from build123d import *

# Parameters (mm, degrees)
SKETCH1_W                      = 125
SKETCH1_H                      = 290
BASE_FLANGE1_DEPTH             = 3.03784
EDGE_FLANGE1_DEPTH             = 290
EDGE_FLANGE1_BEND_DEPTH        = 290
EDGE_FLANGE2_STRIP_W           = 18.50136
EDGE_FLANGE2_STRIP_H           = 3.03784
EDGE_FLANGE2_STRIP_CUT_DEPTH   = 290
EDGE_FLANGE2_STRIP_2_W         = 18.50136
EDGE_FLANGE2_STRIP_2_H         = 3.03784
EDGE_FLANGE2_STRIP_CUT_2_DEPTH = 290
EDGE_FLANGE2_DEPTH             = 290
EDGE_FLANGE2_BEND_DEPTH        = 290
M6_CLEARANCE_HOLE1_D           = 8
CUT_EXTRUDE1_DEPTH             = 50


# Sheet-metal steps are written as plain solids
with BuildPart() as part:
    # Sketch1 → Base-Flange1 (new body)
    with BuildSketch(Plane(origin=(0, 0, 0), x_dir=(0, 0, -1), z_dir=(1, 0, 0))):
        Rectangle(SKETCH1_W, SKETCH1_H)
    extrude(amount=-BASE_FLANGE1_DEPTH)

    # Edge-Flange1 section (across the edge) → Edge-Flange1 (add)
    with BuildSketch(Plane(origin=(-3.03784, -145, 65.675), x_dir=(0, 0, -1), z_dir=(0, 1, 0))):
        with BuildLine():
            Line((-3.03784, 3.175), (-3.03784, 55))
            Line((-3.03784, 55), (0, 55))
            Line((0, 55), (0, 3.175))
            ThreePointArc((0, 3.175), (0.92993597, 0.92993597), (3.175, 0))
            Line((3.175, 0), (3.175, -3.03784))
            ThreePointArc((3.175, -3.03784), (-1.218141294, -1.218141294), (-3.03784, 3.175))
        make_face()
    extrude(amount=EDGE_FLANGE1_DEPTH)

    # Edge-Flange1 section 2 (across the edge) → Edge-Flange1 bend (add)
    with BuildSketch(Plane(origin=(-3.03784, 145, -65.675), x_dir=(0, 0, 1), z_dir=(0, -1, 0))):
        with BuildLine():
            Line((-3.03784, 3.175), (-3.03784, 55))
            Line((-3.03784, 55), (0, 55))
            Line((0, 55), (0, 3.175))
            ThreePointArc((0, 3.175), (0.92993597, 0.92993597), (3.175, 0))
            Line((3.175, 0), (3.175, -3.03784))
            ThreePointArc((3.175, -3.03784), (-1.218141294, -1.218141294), (-3.03784, 3.175))
        make_face()
    extrude(amount=EDGE_FLANGE1_BEND_DEPTH)

    # Edge-Flange2 strip (across the edge) → Edge-Flange2 strip cut (cut)
    with BuildSketch(Plane(origin=(-58.03784, -145, -68.71284), x_dir=(1, 0, 0), z_dir=(0, 1, 0))):
        with Locations((-3.03784, -1.51892)):
            Rectangle(EDGE_FLANGE2_STRIP_W, EDGE_FLANGE2_STRIP_H)
    extrude(amount=EDGE_FLANGE2_STRIP_CUT_DEPTH, mode=Mode.SUBTRACT)

    # Edge-Flange2 strip 2 (across the edge) → Edge-Flange2 strip cut 2 (cut)
    with BuildSketch(Plane(origin=(-58.03784, 145, 68.71284), x_dir=(1, 0, 0), z_dir=(0, -1, 0))):
        with Locations((-3.03784, -1.51892)):
            Rectangle(EDGE_FLANGE2_STRIP_2_W, EDGE_FLANGE2_STRIP_2_H)
    extrude(amount=EDGE_FLANGE2_STRIP_CUT_2_DEPTH, mode=Mode.SUBTRACT)

    # Edge-Flange2 section (across the edge) → Edge-Flange2 (add)
    with BuildSketch(Plane(origin=(-58.03784, -145, -68.71284), x_dir=(1, 0, 0), z_dir=(0, 1, 0))):
        with BuildLine():
            Line((0, 3.175), (0, 30))
            Line((0, 30), (3.03784, 30))
            Line((3.03784, 30), (3.03784, 3.175))
            ThreePointArc((3.03784, 3.175), (3.96777597, 0.92993597), (6.21284, 0))
            Line((6.21284, 0), (6.21284, -3.03784))
            ThreePointArc((6.21284, -3.03784), (1.819698706, -1.218141294), (0, 3.175))
        make_face()
    extrude(amount=EDGE_FLANGE2_DEPTH)

    # Edge-Flange2 section 2 (across the edge) → Edge-Flange2 bend (add)
    with BuildSketch(Plane(origin=(-58.03784, 145, 68.71284), x_dir=(1, 0, 0), z_dir=(0, -1, 0))):
        with BuildLine():
            Line((0, 3.175), (0, 30))
            Line((0, 30), (3.03784, 30))
            Line((3.03784, 30), (3.03784, 3.175))
            ThreePointArc((3.03784, 3.175), (3.96777597, 0.92993597), (6.21284, 0))
            Line((6.21284, 0), (6.21284, -3.03784))
            ThreePointArc((6.21284, -3.03784), (1.819698706, -1.218141294), (0, 3.175))
        make_face()
    extrude(amount=EDGE_FLANGE2_BEND_DEPTH)

    # M6 Clearance Hole1 (through all)
    with Locations(Plane(origin=(-55, 0, 0), x_dir=(0, 0, -1), z_dir=(1, 0, 0))):
        with Locations((-80, 120), (80, 120), (80, -120), (-80, -120)):
            Hole(M6_CLEARANCE_HOLE1_D / 2)

    # Sketch20 → Cut-Extrude1 (cut)
    with BuildSketch(Plane.XY.offset(98.71284)):
        with BuildLine():
            Line((-58.03784, 56.1), (-32.63784, 56.1))
            ThreePointArc((-32.63784, 56.1), (-19.93784, 43.4), (-32.63784, 30.7))
            Line((-32.63784, 30.7), (-58.03784, 30.7))
            Line((-58.03784, 30.7), (-58.03784, 56.1))
        make_face()
    extrude(amount=-CUT_EXTRUDE1_DEPTH, mode=Mode.SUBTRACT)


solid = part.part
Here's how the part is built. I have some questions about the finished solid (model axes, mm). A direction names the side the tool comes from. Coordinates: 2 decimals unless noted, no trailing zeros. Order: outer loops, then holes, each group sorted by start corner. A loop starts at its lowest first (then second) coordinate and runs counter-clockwise, first axis right, second up. Notation, with made-up numbers: (12.25, 59) -> (46.25, 59) arc R30 ccw to (46.25, 98) -> close; hole circle Ø9 at (15.5, 13.25). An arc over 180 degrees is marked (long way). Answer in a Markdown table with one row per item.
(1) I want a section at D-D on z = -80. List the corners of the cut face in (x, y) for me.
Answer key:
| item | result |
|---|---|
| outline | (-58.04, -145) -> (-55, -145) -> (-55, -124) -> (-58.04, -124) -> close; (-58.04, -116) -> (-55, -116) -> (-55, 116) -> (-58.04, 116) -> close; (-58.04, 124) -> (-55, 124) -> (-55, 145) -> (-58.04, 145) -> close |
(2) On a 3-axis mill with a long thin cutter (end or side, diameter ignored), from which of +Z, -Z, +X, -X, +Y, -Y can I reach the whole of each face in a straight line? I mean faces 1 (the face through (-55, 101, 85)), 2 (the face through (-3.038, 2, 1)), 3 (the face through (-56, 30.7, 76)), 4 (the face through (0, 2, 1)), 5 (the face through (-29, 2, -68.713)). Say none if no direction works.
Answer key:
| item | result |
|---|---|
| face 1 | +Z, +X, +Y, -Y |
| face 2 | -X, +Y, -Y |
| face 3 | +Z, -X |
| face 4 | +Z, -Z, +X, +Y, -Y |
| face 5 | -Z, +X, +Y, -Y |
(3) Thinking about a two-plate mould opening in Y: for faces 6 (the face through (-56.54, 123.966, 79.479)), 7 (the face through (-58.038, -56, 85)), 8 (the face through (-1, 145, 30)), which applies, +Y half, -Y half, draft (parallel to the pull), parting line (faces both ways), or undercut?
Answer key:
| item | result |
|---|---|
| face 6 | undercut |
| face 7 | draft |
| face 8 | +Y half |
(4) Will these pins go through, and if not, where does the flat tip stop? pin 1 Ø13.5 at (y, z) = (98, 86.5) entering from +X; pin 2 Ø4 at (x, y) = (-35, 69) entering from -Z; pin 3 Ø10 at (x, z) = (-12, 55.5) entering from -Y; pin 4 Ø23 at (x, y) = (-22, -4) entering from +Z.
Answer key:
| item | result |
|---|---|
| pin 1 | x = -55 |
| pin 2 | z = -68.71 |
| pin 3 | through |
| pin 4 | z = 68.71 |
(5) I want a section at C-C on y = 78. List the corners of the cut face in (x, z) for me (3 decimals), then the cut area to 3 significant figures.
Answer key:
| item | result |
|---|---|
| outline | (-58.038, -98.713) -> (-55, -98.713) -> (-55, -71.888) arc R3.175 cw to (-51.825, -68.713) -> (-6.213, -68.713) arc R6.213 ccw to (0, -62.5) -> (0, 62.5) arc R6.213 ccw to (-6.213, 68.713) -> (-51.825, 68.713) arc R3.175 cw to (-55, 71.888) -> (-55, 98.713) -> (-58.038, 98.713) -> (-58.038, 71.888) arc R6.213 ccw to (-51.825, 65.675) -> (-6.213, 65.675) arc R3.175 cw to (-3.038, 62.5) -> (-3.038, -62.5) arc R3.175 cw to (-6.213, -65.675) -> (-51.825, -65.675) arc R6.213 ccw to (-58.038, -71.888) -> close |
| area | 909 mm^2 |
(6) I want a section at B-B on z = 80. List the corners of the cut face in (x, y) for me.
Answer key:
| item | result |
|---|---|
| outline | (-58.04, -145) -> (-55, -145) -> (-55, -124) -> (-58.04, -124) -> close; (-58.04, -116) -> (-55, -116) -> (-55, 30.7) -> (-58.04, 30.7) -> close; (-58.04, 56.1) -> (-55, 56.1) -> (-55, 116) -> (-58.04, 116) -> close; (-58.04, 124) -> (-55, 124) -> (-55, 145) -> (-58.04, 145) -> close |
(7) I want a section at A-A on y = -120. List the corners of the cut face in (x, z) for me (3 decimals).
Answer key:
| item | result |
|---|---|
| outline | (-58.038, -98.713) -> (-55, -98.713) -> (-55, -84) -> (-58.038, -84) -> close; (-58.038, -76) -> (-55, -76) -> (-55, -71.888) arc R3.175 cw to (-51.825, -68.713) -> (-6.213, -68.713) arc R6.213 ccw to (0, -62.5) -> (0, 62.5) arc R6.213 ccw to (-6.213, 68.713) -> (-51.825, 68.713) arc R3.175 cw to (-55, 71.888) -> (-55, 76) -> (-58.038, 76) -> (-58.038, 71.888) arc R6.213 ccw to (-51.825, 65.675) -> (-6.213, 65.675) arc R3.175 cw to (-3.038, 62.5) -> (-3.038, -62.5) arc R3.175 cw to (-6.213, -65.675) -> (-51.825, -65.675) arc R6.213 ccw to (-58.038, -71.888) -> close; (-58.038, 84) -> (-55, 84) -> (-55, 98.713) -> (-58.038, 98.713) -> close |
(8) Please list where these lines run through material, in increasing order: probe 1 along Y at (x, z) = (-56.4, -80); probe 2 along Z at (x, y) = (-36, 127.5) (3 decimals); probe 3 along X at (y, z) = (-79, 22).
Answer key:
| item | result |
|---|---|
| probe 1 | -145 to -124, -116 to 116, 124 to 145 |
| probe 2 | -68.713 to -65.675, 65.675 to 68.713 |
| probe 3 | -3.04 to 0 |
